Autodesk Inventor part; units mm, degrees
ref_plane "YZ Plane" through (0, 0, 0) normal (1, 0, 0) x (0, 1, 0)
ref_plane "XZ Plane" through (0, 0, 0) normal (0, 1, 0) x (-1, 0, 0)
ref_plane "XY Plane" through (0, 0, 0) normal (0, 0, 1) x (1, 0, 0)
sketch "Sketch1" plane through (0, 0, 0) normal (0, 1, 0) x (-1, 0, 0)
  line L0 (5, 20) -> (-5, 20)
  line L1 (-5, 20) -> (-5, -20)
  line L2 (-5, -20) -> (5, -20)
  line L3 (5, -20) -> (5, 20)
  point P0 (0, 0)
  point P1 (0, -20)
  point P2 (-5, 0)
  dimension "d0" = 10
  dimension "d1" = 40
extrude "Extrusion1" add sketch "Sketch1" along normal blind 4
sketch "Sketch2" plane through (0, 4, 0) normal (0, 1, 0) x (1, 0, 0)
  line L0 (-5, 20) -> (-5, -20)
  line L1 (5, -20) -> (5, 20)
  line L2 (-5, -20) -> (5, -20)
  line L3 (5, -20) -> (5, -7)
  line L4 (5, -7) -> (-5, -7)
  line L5 (-5, -7) -> (-5, -20)
  line L6 (5, 20) -> (-5, 20)
  line L7 (-5, 20) -> (5, 20)
  line L8 (5, 20) -> (5, 7)
  line L9 (5, 7) -> (-5, 7)
  line L10 (-5, 7) -> (-5, 20)
  point P0 (0, 0)
  dimension "d4" = 13
  dimension "d5" = 13
extrude "Extrusion2" add sketch "Sketch2" along normal blind 1.3 contours L6 L1 L9 L0 | L4 L1 L2 L0
sketch "Sketch3" plane through (0, 4, 0) normal (0, 1, 0) x (1, 0, 0)
  point P0 (0, 0)
  point P1 (0, 0)
hole "Hole1" at (0, 4, 0) direction (0, -1, 0) diameter 4.5 end through all
properties part number "Belt Clamp"
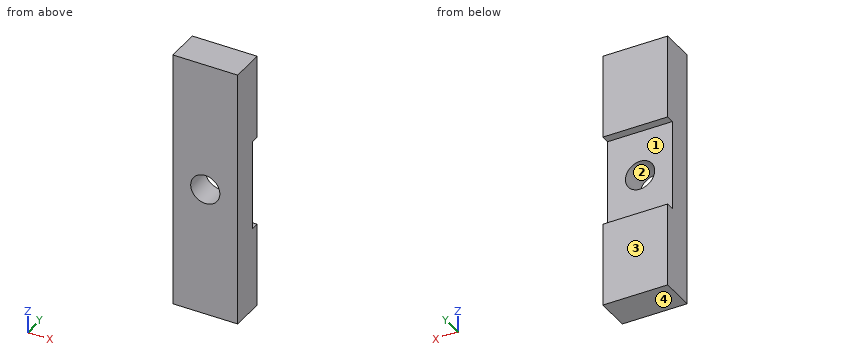
CAD build for the part. Positions are in the model's coordinates, mm. Face numbers are marked on the shaded views. Round coordinates to 2 decimals unless told otherwise and drop trailing zeros. Write each loop counter-clockwise with the first axis right and the second up, starting at its lowest first coordinate (ties: lowest second). Pieces come first, ordered by that corner, then holes.
Item 1: Band-saw the part on A-A on z = 0. Write the cut outline in (x, y), then the cut area to 3 significant figures.
Filled in:
outline: (-5, 0) - (-2.25, 0) - (-2.25, 4) - (-5, 4) - close; (2.25, 0) - (5, 0) - (5, 4) - (2.25, 4) - close
area: 22.0 mm2
Item 2: Drop a flat-ended pin along its axis: pin 1 Ø5 at (x, z) = (2.5, -2.5) entering from +Y. Give the stop position or say it passes through.
Filled in:
pin 1: stops at y = 4
Item 3: Drill centre lines: L1, parallel to Z at x = 1, y = 4.05; L2, parallel to X at y = 1, z = 0; L3, parallel to Z at x = 0, y = 0.8. Where is each one in solid material? Low to high.
Filled in:
L1: z = -20 to -7, 7 to 20
L2: x = -5 to -2.25, 2.25 to 5
L3: z = -20 to -2.25, 2.25 to 20
Item 4: Band-saw the part on B-B on x = 0. Write the cut outline in (y, z), then the cut area to 3 significant figures.
Filled in:
outline: (0, -20) - (5.3, -20) - (5.3, -7) - (4, -7) - (4, -2.25) - (0, -2.25) - close; (0, 2.25) - (4, 2.25) - (4, 7) - (5.3, 7) - (5.3, 20) - (0, 20) - close
area: 176 mm2
Item 5: Band-saw the part on D-D on x = 4. Write the cut outline in (y, z).
Filled in:
outline: (0, -20) - (5.3, -20) - (5.3, -7) - (4, -7) - (4, 7) - (5.3, 7) - (5.3, 20) - (0, 20) - close
Item 6: Mould opens along Z. For the marked faces 1, 2, 3 and 4 say: released by +Z, released by -Z, zero draft, split by the parting line, or undercut.
Filled in:
face 1: undercut
face 2: undercut
face 3: zero draft
face 4: released by -Z
Item 7: Band-saw the part on C-C on y = 4.65. Write the cut outline in (x, z), then the cut area to 3 significant figures.
Filled in:
outline: (-5, -20) - (5, -20) - (5, -7) - (-5, -7) - close; (-5, 7) - (5, 7) - (5, 20) - (-5, 20) - close
area: 260 mm2
